Can you work these out from the model? Positions are in its coordinate system, mm. A direction names the side the tool comes from. Coordinates: 2 decimals unless noted, no trailing zeros. Write each loop counter-clockwise with the first axis right and the second up, starting at its lowest first coordinate (ties: lowest second). Pieces come first, ordered by that corner, then holes. Notation, with made-up numbers: (-19.75, 75) - (39.25, 75) arc R9 ccw to (39.25, 84) - close; hole circle Ø10 at (52.5, 6.25). An arc over 180 degrees is marked (long way). Use one line per item in the form item = value. Start each with the question number.
(1) If we section it at C-C on z = -6.25: Please give me the cut outline in (x, y), then the cut area to 3 significant figures.
(2) If we section it at B-B on x = 3.5: Please give me the cut outline in (y, z), then the cut area to 3 significant figures.
(3) If I drill on probe 1 along X at (y, z) = (0.2, -6.25); probe 2 along Z at (x, y) = (-3.5, 1.35); probe 3 along X at (y, z) = (0.55, -18), over which ranges is the centre line in solid material (lowest first)? Write a range as from..to.
(4) Thinking about a two-plate mould opening in X: for faces 1 (the face through (0, 1, -21)), 2 (the face through (12, 0.484, -6)), 3 (the face through (4, 0, 7)), 4 (the face through (-0.34, 1, 14.05)), which applies, pulls with the +X half, pulls with the -X half, needs draft (parallel to the pull), parting line crosses it, or undercut?
(5) On a 3-axis mill with a long thin cutter (end or side, diameter ignored), from which of +Z, -Z, +X, -X, +Y, -Y can I reach the whole of each face in a straight line? I mean faces 5 (the face through (11.53, 0.24, -5.71)), 6 (the face through (-9.311, 0.999, -6.727)). Say none if no direction works.
(6) For pin 1 Ø1 at (x, z) = (-11.5, -7) entering from +Y, with a flat end and sliding along its axis, tell me the tip position at first contact or that it passes through.
(7) If we section it at D-D on z = -0.5: Please give me the cut outline in (x, y), then the cut area to 3 significant figures.
(8) If we section it at A-A on y = 0.9: Give the number of separate pieces and of enclosed holes in the cut face, then the cut area to 3 significant figures.
```python
from build123d import *

# Parameters (mm, degrees)
BOSS_EXTRUDE1_DEPTH                            = 1.5
CBORE_FOR_0_SOCKET_HEAD_CAP_SCREW1_D           = 1.778
CBORE_FOR_0_SOCKET_HEAD_CAP_SCREW1_CBORE_D     = 3.175
CBORE_FOR_0_SOCKET_HEAD_CAP_SCREW1_CBORE_DEPTH = 1.016


with BuildPart() as part:
    # Sketch1 → Boss-Extrude1 (new body)
    with BuildSketch(Plane(origin=(0, 0, 0), x_dir=(1, 0, 0), z_dir=(0, 1, 0))):
        with BuildLine():
            ThreePointArc((-15.564231563, -8.000293485), (-16.028200148, -7.024727753), (-16.431091722, -6.022393613))
            Line((-16.431091722, -6.022393613), (-17.088457268, -6.401923789))
            ThreePointArc((-17.088457268, -6.401923789), (-18.186533479, -10.5), (-14.088457268, -11.598076211))
            Line((-14.088457268, -11.598076211), (-13.431091722, -11.218546036))
            ThreePointArc((-13.431091722, -11.218546036), (-14.097692763, -10.368464629), (-14.710573178, -9.478873181))
            ThreePointArc((-14.710573178, -9.478873181), (-16.454482672, -9.5), (-15.564231563, -8.000293485))
        make_face()
        with BuildLine():
            ThreePointArc((-7.45294045, -0.83885556), (-6.495190528, 3.75), (-3, 6.873863542))
            Line((-3, 6.873863542), (-3, 17.24093965))
            ThreePointArc((-3, 17.24093965), (-15.155444566, 8.75), (-16.431091722, -6.022393613))
            Line((-16.431091722, -6.022393613), (-7.45294045, -0.83885556))
        make_face()
        with BuildLine():
            ThreePointArc((-4.45294045, -6.035007983), (-6.495190528, -3.75), (-7.45294045, -0.83885556))
            Line((-7.45294045, -0.83885556), (-16.431091722, -6.022393613))
            ThreePointArc((-16.431091722, -6.022393613), (-16.028200148, -7.024727753), (-15.564231563, -8.000293485))
            ThreePointArc((-15.564231563, -8.000293485), (-14.872836662, -8.301510811), (-14.588457268, -9))
            ThreePointArc((-14.588457268, -9), (-14.619467049, -9.247099079), (-14.710573178, -9.478873181))
            ThreePointArc((-14.710573178, -9.478873181), (-14.097692763, -10.368464629), (-13.431091722, -11.218546036))
            Line((-13.431091722, -11.218546036), (-4.45294045, -6.035007983))
        make_face()
        with BuildLine():
            ThreePointArc((4.45294045, -6.035007983), (0, -7.5), (-4.45294045, -6.035007983))
            Line((-4.45294045, -6.035007983), (-13.431091722, -11.218546036))
            ThreePointArc((-13.431091722, -11.218546036), (0, -17.5), (13.431091722, -11.218546036))
            Line((13.431091722, -11.218546036), (4.45294045, -6.035007983))
        make_face()
        with BuildLine():
            ThreePointArc((7.45294045, -0.83885556), (6.495190528, -3.75), (4.45294045, -6.035007983))
            Line((4.45294045, -6.035007983), (13.431091722, -11.218546036))
            ThreePointArc((13.431091722, -11.218546036), (14.097692763, -10.368464629), (14.710573178, -9.478873181))
            ThreePointArc((14.710573178, -9.478873181), (14.722431864, -8.5), (15.564231563, -8.000293485))
            ThreePointArc((15.564231563, -8.000293485), (16.028200148, -7.024727753), (16.431091722, -6.022393613))
            Line((16.431091722, -6.022393613), (7.45294045, -0.83885556))
        make_face()
        with BuildLine():
            Line((3, 17.24093965), (3, 6.873863542))
            ThreePointArc((3, 6.873863542), (6.274950199, 4.107919181), (7.5, 0))
            ThreePointArc((7.5, 0), (7.48822587, -0.420087268), (7.45294045, -0.83885556))
            Line((7.45294045, -0.83885556), (16.431091722, -6.022393613))
            ThreePointArc((16.431091722, -6.022393613), (17.230700873, -3.05825889), (17.5, 0))
            ThreePointArc((17.5, 0), (13.393095236, 11.263880326), (3, 17.24093965))
        make_face()
        with BuildLine():
            Line((-3, 18), (-3, 17.24093965))
            ThreePointArc((-3, 17.24093965), (-1.930507386, 17.393192382), (-0.853658385, 17.479166667))
            ThreePointArc((-0.853658385, 17.479166667), (-0.27050103, 18.962719685), (1, 18))
            ThreePointArc((1, 18), (0.962719685, 17.72949897), (0.853658385, 17.479166667))
            ThreePointArc((0.853658385, 17.479166667), (1.930507386, 17.393192382), (3, 17.24093965))
            Line((3, 17.24093965), (3, 18))
            ThreePointArc((3, 18), (0, 21), (-3, 18))
        make_face()
        with BuildLine():
            Line((-3, 17.24093965), (-3, 6.873863542))
            ThreePointArc((-3, 6.873863542), (0, 7.5), (3, 6.873863542))
            Line((3, 6.873863542), (3, 17.24093965))
            ThreePointArc((3, 17.24093965), (1.930507386, 17.393192382), (0.853658385, 17.479166667))
            ThreePointArc((0.853658385, 17.479166667), (0, 17), (-0.853658385, 17.479166667))
            ThreePointArc((-0.853658385, 17.479166667), (-1.930507386, 17.393192382), (-3, 17.24093965))
        make_face()
        with BuildLine():
            ThreePointArc((14.710573178, -9.478873181), (14.097692763, -10.368464629), (13.431091722, -11.218546036))
            Line((13.431091722, -11.218546036), (14.088457268, -11.598076211))
            ThreePointArc((14.088457268, -11.598076211), (18.186533479, -10.5), (17.088457268, -6.401923789))
            Line((17.088457268, -6.401923789), (16.431091722, -6.022393613))
            ThreePointArc((16.431091722, -6.022393613), (16.028200148, -7.024727753), (15.564231563, -8.000293485))
            ThreePointArc((15.564231563, -8.000293485), (16.286946457, -8.284379393), (16.588457268, -9))
            ThreePointArc((16.588457268, -9), (15.835556347, -9.968990219), (14.710573178, -9.478873181))
        make_face()
    extrude(amount=BOSS_EXTRUDE1_DEPTH)

    # CBORE for #0 Socket Head Cap Screw1 (through all)
    with Locations(Plane(origin=(0, 1.5, 0), x_dir=(1, 0, 0), z_dir=(0, 1, 0))):
        with Locations((-10.825317547, 6.25), (10.825317547, 6.25), (0, -12.5)):
            CounterBoreHole(CBORE_FOR_0_SOCKET_HEAD_CAP_SCREW1_D / 2, CBORE_FOR_0_SOCKET_HEAD_CAP_SCREW1_CBORE_D / 2, CBORE_FOR_0_SOCKET_HEAD_CAP_SCREW1_CBORE_DEPTH)


solid = part.part
```
Reported:
q1.outline = (-16.35, 0) - (-11.71, 0) - (-11.71, 0.48) - (-12.41, 0.48) - (-12.41, 1.5) - (-16.35, 1.5) - close; (-9.94, 0) - (-4.15, 0) - (-4.15, 1.5) - (-9.24, 1.5) - (-9.24, 0.48) - (-9.94, 0.48) - close; (4.15, 0) - (9.94, 0) - (9.94, 0.48) - (9.24, 0.48) - (9.24, 1.5) - (4.15, 1.5) - close; (11.71, 0) - (16.35, 0) - (16.35, 1.5) - (12.41, 1.5) - (12.41, 0.48) - (11.71, 0.48) - close
q1.area = 28.4 mm2
q2.outline = (0, -17.15) - (1.5, -17.15) - (1.5, -6.63) - (0, -6.63) - close; (0, 6.63) - (1.5, 6.63) - (1.5, 17.15) - (0, 17.15) - close
q2.area = 31.5 mm2
q3.probe_1 = -16.35..-11.71, -9.94..-4.15, 4.15..9.94, 11.71..16.35
q3.probe_2 = -17.15..-6.63, 6.63..17.15
q3.probe_3 = -3..-1, 1..3
q4.face_1 = parting line crosses it
q4.face_2 = undercut
q4.face_3 = needs draft
q4.face_4 = undercut
q5.face_5 = +Y, -Y
q5.face_6 = +Y
q6.pin_1 = 0.48
q7.outline = (-17.49, 0) - (-7.48, 0) - (-7.48, 1.5) - (-17.49, 1.5) - close; (7.48, 0) - (17.49, 0) - (17.49, 1.5) - (7.48, 1.5) - close
q7.area = 30.0 mm2
q8.separate_pieces = 1
q8.enclosed_holes = 7
q8.area = 805 mm2
